```python
from build123d import *

# Parameters (mm, degrees)
SKETCH1_R               = 16
BOSS_EXTRUDE1_DEPTH     = 3
SKETCH2_R               = 8
SKETCH2_R_2             = 3
BOSS_EXTRUDE2_DEPTH     = 10
SKETCH3_R               = 2
CUT_EXTRUDE1_DEPTH      = 25.738633754
CUT_EXTRUDE2_DEPTH      = 27.095976701
CUT_EXTRUDE2_DEPTH_BACK = 27.095976701
SKETCH4_R               = 2


with BuildPart() as part:
    # Sketch1 → Boss-Extrude1 (new body)
    with BuildSketch(Plane.XY):
        Circle(SKETCH1_R)
    extrude(amount=BOSS_EXTRUDE1_DEPTH)

    # Sketch2 → Boss-Extrude2 (add)
    with BuildSketch(Plane.XY.offset(3)):
        Circle(SKETCH2_R)
        Circle(SKETCH2_R_2, mode=Mode.SUBTRACT)
    extrude(amount=BOSS_EXTRUDE2_DEPTH)

    # Sketch3 → Cut-Extrude1 (cut, through all)
    with BuildSketch(Plane.XY.offset(3)):
        with Locations((0, 12)):
            Circle(SKETCH3_R)
        with Locations((12, 0)):
            Circle(SKETCH3_R)
        with Locations((0, -12)):
            Circle(SKETCH3_R)
        with Locations((-12, 0)):
            Circle(SKETCH3_R)
    extrude(amount=-CUT_EXTRUDE1_DEPTH, mode=Mode.SUBTRACT)

    # Sketch4 → Cut-Extrude2 (cut, two sides: drawn at the far end of the back side and taken through both)
    with BuildSketch(Plane(origin=(0, 0, 0), x_dir=(1, 0, 0), z_dir=(0, 1, 0)).offset(-CUT_EXTRUDE2_DEPTH_BACK)):
        with Locations(Location((0, -8, 0), (0, 0, 270))):
            Circle(SKETCH4_R)
    extrude(amount=CUT_EXTRUDE2_DEPTH + CUT_EXTRUDE2_DEPTH_BACK, mode=Mode.SUBTRACT)


solid = part.part
```
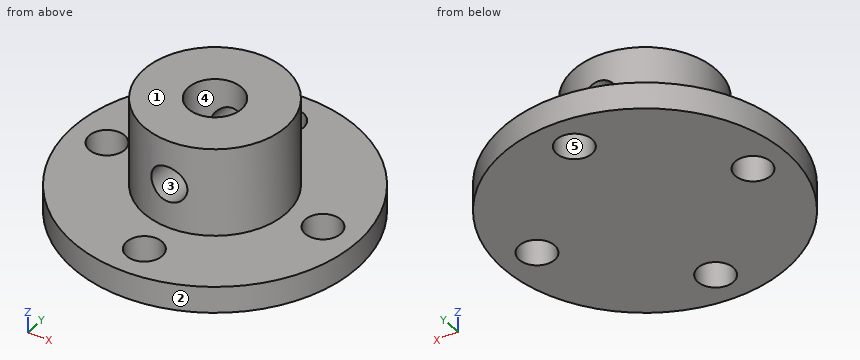
For this review, take the finished solid that the model builds, in its own axes (mm). Face numbers are marked on the shaded views. A direction names the side the tool comes from. Round coordinates to 2 decimals unless told otherwise and drop trailing zeros. Order: outer loops, then holes, each group sorted by start corner. A loop starts at its lowest first (then second) coordinate and runs counter-clockwise, first axis right, second up.
Q1. Insertion check: P1, Ø6.5, axis at x = 0, z = 8, coming from the +Y side; P2, Ø6.5, axis at x = 0, y = -12, coming from the +Z side; P3, Ø5, axis at x = 3.5, z = 3.5, coming from the +Y side; P4, Ø2.5, axis at x = 0, y = 12, coming from the -Z side. Each pin has a flat end and moves straight along its axis. Give the tip position at first contact, or say it passes through.
Findings below:
P1: stops at y = 8
P2: stops at z = 3
P3: stops at y = 15.97
P4: passes through
Q2. We need section B-B, the plane y = 0. Give the boundary of the cut face in (x, z).
Findings below:
outline: (-16, 0) - (-14, 0) - (-14, 3) - (-16, 3) - close; (-10, 0) - (10, 0) - (10, 3) - (8, 3) - (8, 13) - (3, 13) - (3, 3) - (-3, 3) - (-3, 13) - (-8, 13) - (-8, 3) - (-10, 3) - close; (14, 0) - (16, 0) - (16, 3) - (14, 3) - close
Q3. We need section D-D, the plane x = -12. Give the boundary of the cut face in (y, z), plus the area to 3 significant figures.
Findings below:
outline: (-10.58, 0) - (-2, 0) - (-2, 3) - (-10.58, 3) - close; (2, 0) - (10.58, 0) - (10.58, 3) - (2, 3) - close
area: 51.5 mm2
Q4. Machinability: for the marked faces 4 and 5, which of the approach directions +Z, -Z, +X, -X, +Y, -Y give a long, thin tool a straight path to every point of the face, cutting with its end or side? Answer none if there is none.
Findings below:
face 4: +Z
face 5: +Z, -Z
Q5. We need section C-C, the plane z = 7.25. Give the boundary of the cut face in (x, y).
Findings below:
outline: (-1.85, -7.78) - (-1.85, -2.36) arc R3 cw to (-1.85, 2.36) - (-1.85, 7.78) arc R8 ccw to start; (1.85, -7.78) arc R8 ccw to (1.85, 7.78) - (1.85, 2.36) arc R3 cw to (1.85, -2.36) - close
Q6. Wall thickness on line 1 (Y direction, x = 0, z = 2.1); line 2 (X direction, y = -5, z = 7.5) (1 decimal); line 3 (Z direction, x = -9, y = -9.5): over which ranges is each line inside the solid? List them lowest first.
Findings below:
line 1: y = -16 to -14, -10 to 10, 14 to 16
line 2: x = -6.2 to -1.9, 1.9 to 6.2
line 3: z = 0 to 3
Q7. We need section A-A, the plane x = 0. Give the boundary of the cut face in (y, z), plus the area to 3 significant figures.
Findings below:
outline: (-16, 0) - (-14, 0) - (-14, 3) - (-16, 3) - close; (-10, 0) - (10, 0) - (10, 3) - (8, 3) - (8, 6) - (3, 6) - (3, 3) - (-3, 3) - (-3, 6) - (-8, 6) - (-8, 3) - (-10, 3) - close; (-8, 10) - (-3, 10) - (-3, 13) - (-8, 13) - close; (3, 10) - (8, 10) - (8, 13) - (3, 13) - close; (14, 0) - (16, 0) - (16, 3) - (14, 3) - close
area: 132 mm2
Q8. Mouldability with a two-part tool opening along X and no side actions: class the marked faces 1, 2 and 3 as pulls with the +X half, pulls with the -X half, needs draft (parallel to the pull), parting line crosses it, or undercut.
Findings below:
face 1: needs draft
face 2: parting line crosses it
face 3: undercut
